from build123d import *

# Parameters (mm, degrees)
F0_R     = 14
F1_DEPTH = 8


with BuildPart() as f1:
    # F0 (on Top) → F1 (new body)
    with BuildSketch(Plane.XY):
        with BuildLine():
            ThreePointArc((57, -5.196152), (32.842323, 18.961524), (24, 51.961524))
            ThreePointArc((24, 51.961524), (0, 75.961524), (-24, 51.961524))
            ThreePointArc((-24, 51.961524), (-32.842323, 18.961524), (-57, -5.196152))
            ThreePointArc((-57, -5.196152), (-65.78461, -37.980762), (-33, -46.765372))
            ThreePointArc((-33, -46.765372), (0, -37.923048), (33, -46.765372))
            ThreePointArc((33, -46.765372), (65.78461, -37.980762), (57, -5.196152))
        make_face()
        with Locations((-45, -25.980762)):
            Circle(F0_R, mode=Mode.SUBTRACT)
        Circle(F0_R, mode=Mode.SUBTRACT)
        with Locations((45, -25.980762)):
            Circle(F0_R, mode=Mode.SUBTRACT)
        with Locations((0, 51.961524)):
            Circle(F0_R, mode=Mode.SUBTRACT)
    extrude(amount=F1_DEPTH)


solid = f1.part
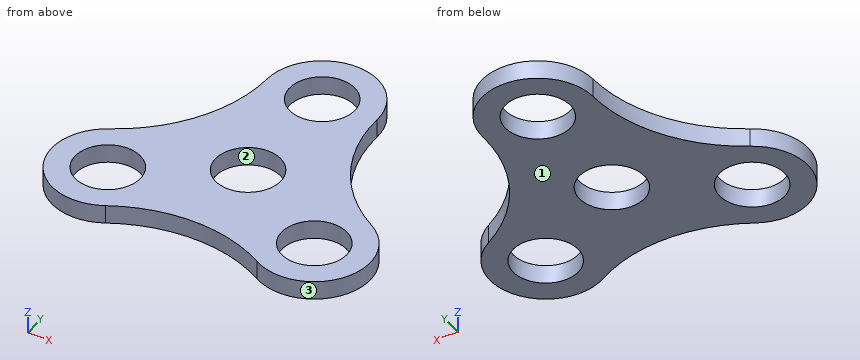
Here's how the part is built. I have some questions about the finished solid (model axes, mm). Face numbers are marked on the shaded views. Round coordinates to 2 decimals unless told otherwise and drop trailing zeros. Order: outer loops, then holes, each group sorted by start corner. A loop starts at its lowest first (then second) coordinate and runs counter-clockwise, first axis right, second up. Notation, with made-up numbers: M -39,22.5 L 12,22.5 A19 cw 12,45.5 Z; hole C -23.5,11.25 d5. An arc over 180 degrees is marked long. Return JSON: item names as keys, results as strings. Group by question number.
1. If we section it at D-D on x = 45: List the corners of the cut face in (y, z) for me.
2. If we section it at B-B on y = 0: List the corners of the cut face in (x, z) for me, then the cut area to 3 significant figures.
3. If we mould it in two halves opening along Y, with no side actions, what happens to the marked faces 1, 2 and 3? For each: pulls with the +Y half, pulls with the -Y half, needs draft (parallel to the pull), parting line crosses it, or undercut.
4. If we section it at C-C on z = 1.75: List the corners of the cut face in (x, y) for me, then the cut area to 3 significant figures.
5. Please list where these lines run through material, in increasing order: probe 1 along Y at (x, z) = (0, 3.5); probe 2 along X at (y, z) = (-34, 3.25); probe 3 along X at (y, z) = (-21, 6.75).
6. If we section it at A-A on x = 0: List the corners of the cut face in (y, z) for me, then the cut area to 3 significant figures.
7. I'm going to push flat-ended pins straight in: pin 1 Ø1.5 at (y, z) = (14.5, 1.5) entering from +X; pin 2 Ø1.5 at (y, z) = (34.5, 7) entering from +X; pin 3 Ø2 at (y, z) = (51.5, 2.5) entering from -X. Where does each tip first touch, or does it pass through?
Reply:
{
 "1": {"outline": "M -49.98,0 L -39.98,0 L -39.98,8 L -49.98,8 Z; M -11.98,0 L 3.68,0 L 3.68,8 L -11.98,8 Z"},
 "2": {"outline": "M -49.31,0 L -14,0 L -14,8 L -49.31,8 Z; M 14,0 L 49.31,0 L 49.31,8 L 14,8 Z", "area": "565 mm^2"},
 "3": {"face 1": "needs draft", "face 2": "undercut", "face 3": "parting line crosses it"},
 "4": {"outline": "M -57,-5.2 A24 ccw -33,-46.77 A66 cw 33,-46.77 A24 ccw 57,-5.2 A66 cw 24,51.96 A24 ccw -24,51.96 A66 cw Z; hole C -45,-25.98 d28; hole C 0,0 d28; hole C 0,51.96 d28; hole C 45,-25.98 d28", "area": "7,440 mm^2"},
 "5": {"probe 1": "-37.92 to -14, 14 to 37.96, 65.96 to 75.96", "probe 2": "-67.62 to -56.48, -33.52 to 33.52, 56.48 to 67.62", "probe 3": "-68.48 to -58.08, -31.92 to 31.92, 58.08 to 68.48"},
 "6": {"outline": "M -37.92,0 L -14,0 L -14,8 L -37.92,8 Z; M 14,0 L 37.96,0 L 37.96,8 L 14,8 Z; M 65.96,0 L 75.96,0 L 75.96,8 L 65.96,8 Z", "area": "463 mm^2"},
 "7": {"pin 1": "x = 36.19", "pin 2": "x = 26.56", "pin 3": "x = -24.02"}
}
